```python
from build123d import *

# Parameters (mm, degrees)
SKETCH_1_R          = 1.7
SKETCH_1_R_2        = 2.5
EXTRUDE_1_DEPTH     = 3
SKETCH_2_R          = 2
CUT_EXTRUDE_1_DEPTH = 3


with BuildPart() as part:
    # 草图1 → 凸台-拉伸1 (new body)
    with BuildSketch(Plane(origin=(0, 0, 0), x_dir=(1, 0, 0), z_dir=(0, 1, 0))):
        with BuildLine():
            ThreePointArc((-65, 120), (-68.535533906, 118.535533906), (-70, 115))
            Line((-70, 115), (-70, -115))
            ThreePointArc((-70, -115), (-68.535533906, -118.535533906), (-65, -120))
            Line((-65, -120), (65, -120))
            ThreePointArc((65, -120), (68.535533906, -118.535533906), (70, -115))
            Line((70, -115), (70, 115))
            ThreePointArc((70, 115), (68.535533906, 118.535533906), (65, 120))
            Line((65, 120), (-65, 120))
        make_face()
        with BuildLine():
            Line((-25, 95), (-25, 105))
            ThreePointArc((-25, 105), (-22.071067812, 112.071067812), (-15, 115))
            Line((-15, 115), (15, 115))
            ThreePointArc((15, 115), (22.071067812, 112.071067812), (25, 105))
            Line((25, 105), (25, 95))
            ThreePointArc((25, 95), (22.071067812, 87.928932188), (15, 85))
            Line((15, 85), (-15, 85))
            ThreePointArc((-15, 85), (-22.071067812, 87.928932188), (-25, 95))
        make_face(mode=Mode.SUBTRACT)
        with Locations(Location((-48, 92, 0), (0, 0, 270))):
            Circle(SKETCH_1_R, mode=Mode.SUBTRACT)
        with Locations(Location((-62, 92, 0), (0, 0, 270))):
            Circle(SKETCH_1_R, mode=Mode.SUBTRACT)
        with Locations(Location((-35, 110, 0), (0, 0, 270))):
            Circle(SKETCH_1_R_2, mode=Mode.SUBTRACT)
        with Locations(Location((-48, 108, 0), (0, 0, 270))):
            Circle(SKETCH_1_R, mode=Mode.SUBTRACT)
        with Locations(Location((-62, 108, 0), (0, 0, 270))):
            Circle(SKETCH_1_R, mode=Mode.SUBTRACT)
        with Locations(Location((35, 110, 0), (0, 0, 270))):
            Circle(SKETCH_1_R_2, mode=Mode.SUBTRACT)
        with Locations(Location((62, 108, 0), (0, 0, 270))):
            Circle(SKETCH_1_R, mode=Mode.SUBTRACT)
        with Locations(Location((62, 92, 0), (0, 0, 270))):
            Circle(SKETCH_1_R, mode=Mode.SUBTRACT)
        with Locations(Location((48, 108, 0), (0, 0, 270))):
            Circle(SKETCH_1_R, mode=Mode.SUBTRACT)
        with Locations(Location((-62, -108, 0), (0, 0, 270))):
            Circle(SKETCH_1_R, mode=Mode.SUBTRACT)
        with Locations(Location((-62, -92, 0), (0, 0, 270))):
            Circle(SKETCH_1_R, mode=Mode.SUBTRACT)
        with Locations(Location((-48, -108, 0), (0, 0, 270))):
            Circle(SKETCH_1_R, mode=Mode.SUBTRACT)
        with Locations(Location((-35, -110, 0), (0, 0, 270))):
            Circle(SKETCH_1_R_2, mode=Mode.SUBTRACT)
        with Locations(Location((-48, -92, 0), (0, 0, 270))):
            Circle(SKETCH_1_R, mode=Mode.SUBTRACT)
        with BuildLine():
            ThreePointArc((15, -85), (22.071067812, -87.928932188), (25, -95))
            Line((25, -95), (25, -105))
            ThreePointArc((25, -105), (22.071067812, -112.071067812), (15, -115))
            Line((15, -115), (-15, -115))
            ThreePointArc((-15, -115), (-22.071067812, -112.071067812), (-25, -105))
            Line((-25, -105), (-25, -95))
            ThreePointArc((-25, -95), (-22.071067812, -87.928932188), (-15, -85))
            Line((-15, -85), (15, -85))
        make_face(mode=Mode.SUBTRACT)
        with Locations(Location((35, -110, 0), (0, 0, 270))):
            Circle(SKETCH_1_R_2, mode=Mode.SUBTRACT)
        with Locations(Location((48, -108, 0), (0, 0, 270))):
            Circle(SKETCH_1_R, mode=Mode.SUBTRACT)
        with Locations(Location((48, -92, 0), (0, 0, 270))):
            Circle(SKETCH_1_R, mode=Mode.SUBTRACT)
        with Locations(Location((62, -108, 0), (0, 0, 270))):
            Circle(SKETCH_1_R, mode=Mode.SUBTRACT)
        with Locations(Location((62, -92, 0), (0, 0, 270))):
            Circle(SKETCH_1_R, mode=Mode.SUBTRACT)
        with Locations(Location((48, 92, 0), (0, 0, 270))):
            Circle(SKETCH_1_R, mode=Mode.SUBTRACT)
    extrude(amount=EXTRUDE_1_DEPTH)

    # 草图2 → 切除-拉伸1 (cut)
    with BuildSketch(Plane(origin=(0, 3, 0), x_dir=(1, 0, 0), z_dir=(0, 1, 0))):
        with Locations(Location((-60, 0, 0), (0, 0, 270))):
            Circle(SKETCH_2_R)
        with Locations(Location((-60, 40, 0), (0, 0, 270))):
            Circle(SKETCH_2_R)
        with Locations(Location((-60, 80, 0), (0, 0, 270))):
            Circle(SKETCH_2_R)
        with Locations(Location((-60, -80, 0), (0, 0, 270))):
            Circle(SKETCH_2_R)
        with Locations(Location((-60, -40, 0), (0, 0, 270))):
            Circle(SKETCH_2_R)
        with Locations(Location((-30, 40, 0), (0, 0, 270))):
            Circle(SKETCH_2_R)
        with Locations(Location((-30, 80, 0), (0, 0, 270))):
            Circle(SKETCH_2_R)
        with Locations(Location((-30, -40, 0), (0, 0, 270))):
            Circle(SKETCH_2_R)
        with Locations(Location((-30, -80, 0), (0, 0, 270))):
            Circle(SKETCH_2_R)
        with Locations(Location((30, -80, 0), (0, 0, 270))):
            Circle(SKETCH_2_R)
        with Locations(Location((30, -40, 0), (0, 0, 270))):
            Circle(SKETCH_2_R)
        with Locations(Location((30, 80, 0), (0, 0, 270))):
            Circle(SKETCH_2_R)
        with Locations(Location((30, 40, 0), (0, 0, 270))):
            Circle(SKETCH_2_R)
        with Locations(Location((60, -40, 0), (0, 0, 270))):
            Circle(SKETCH_2_R)
        with Locations(Location((60, -80, 0), (0, 0, 270))):
            Circle(SKETCH_2_R)
        with Locations(Location((60, 80, 0), (0, 0, 270))):
            Circle(SKETCH_2_R)
        with Locations(Location((60, 40, 0), (0, 0, 270))):
            Circle(SKETCH_2_R)
        with Locations(Location((60, 0, 0), (0, 0, 270))):
            Circle(SKETCH_2_R)
        with Locations(Location((0, -40, 0), (0, 0, 270))):
            Circle(SKETCH_2_R)
        with Locations(Location((0, -80, 0), (0, 0, 270))):
            Circle(SKETCH_2_R)
        with Locations(Location((0, 80, 0), (0, 0, 270))):
            Circle(SKETCH_2_R)
        with Locations(Location((0, 40, 0), (0, 0, 90))):
            Circle(SKETCH_2_R)
    extrude(amount=-CUT_EXTRUDE_1_DEPTH, mode=Mode.SUBTRACT)


solid = part.part
```
Input: part model. Units: mm. Frame: model coordinates. A direction names the side the tool comes from. Round coordinates to 2 decimals unless told otherwise and drop trailing zeros. Order: outer loops, then holes, each group sorted by start corner. A loop starts at its lowest first (then second) coordinate and runs counter-clockwise, first axis right, second up. Notation, with made-up numbers: (-13, 33.25) - (37, 33.25) arc R16 cw to (37, 40.25) - close; hole circle Ø4 at (38.5, -20.5). An arc over 180 degrees is marked (long way). One line per question, with ' | ' between items. Start each with the question number.
1) Contact query for a flat-ended pin moving along its axis: P1, Ø2.5, axis at x = 30, z = 40, coming from the -Y side. Output: stop coordinate, or through.
2) Pull-direction query (X, two-part tool) for faces 3 (the flat face through (-1, 0, -2)), 4 (the cylindrical face through (-21.99, 1.48, -87.85)), 5 (the cylindrical face through (35.751, 1.479, -107.615)), 6 (the cylindrical face through (69, 1, -118)); classes: +X half, -X half, draft (parallel to the pull), parting line (faces both ways), or undercut.
3) Ray query, probe 1 along Z at (x, y) = (10, 2.4); probe 2 along X at (y, z) = (0.7, -80); probe 3 along Z at (x, y) = (47, 1.7). Return the intervals inside material, ascending.
4) Cut plane B-B, the plane y = 0.9. Give the number of separate pieces and of enclosed holes in the cut face, then the cut area to 4 significant figures.
5) Cut plane C-C, the plane x = -35. Return the cut outline in (y, z).
6) Set-up query: faces 1 (the cylindrical face through (-22.15, 1.48, -111.99)), 2 (the cylindrical face through (-68, 1, -119)). Return all of +Z, -Z, +X, -X, +Y, -Y with unobstructed straight access to the full face (end or side cutting, diameter ignored); none if empty.
7) Cut plane A-A, the plane x = 11.5. Return the cut outline in (y, z), then the cut area to 3 significant figures.
Worked out:
1) P1: passes through
2) face 3: draft | face 4: undercut | face 5: undercut | face 6: +X half
3) probe 1: z = -120 to -115, -85 to 85, 115 to 120 | probe 2: x = -70 to -62, -58 to -32, -28 to -2, 2 to 28, 32 to 58, 62 to 70 | probe 3: z = -120 to -109.37, -106.63 to -93.37, -90.63 to 90.63, 93.37 to 106.63, 109.37 to 120
4) separate pieces: 1 | enclosed holes: 44 | area: 30,250 mm^2
5) outline: (0, -120) - (3, -120) - (3, -112.5) - (0, -112.5) - close; (0, -107.5) - (3, -107.5) - (3, 107.5) - (0, 107.5) - close; (0, 112.5) - (3, 112.5) - (3, 120) - (0, 120) - close
6) face 1: +Y, -Y | face 2: -Z, -X, +Y, -Y
7) outline: (0, -120) - (3, -120) - (3, -115) - (0, -115) - close; (0, -85) - (3, -85) - (3, 85) - (0, 85) - close; (0, 115) - (3, 115) - (3, 120) - (0, 120) - close | area: 540 mm^2
